Geometry check sheet. Reference: the model listing, model coordinates, mm. A direction names the side the tool comes from. Coordinates: 2 decimals unless noted, no trailing zeros. Order: outer loops, then holes, each group sorted by start corner. A loop starts at its lowest first (then second) coordinate and runs counter-clockwise, first axis right, second up. Notation, with made-up numbers: (59, 38) - (104, 38) arc R20 cw to (104, 55) - close; hole circle Ø6 at (-24, -33). An arc over 180 degrees is marked (long way). Use CSV: the item, a comma, the result in double quotes. Start each with the question number.
1) Sectioned sample at D-D, the plane y = -15. Record the cut outline in (x, z), and give its area (3 significant figures).
2) Sectioned sample at C-C, the plane y = -8. Record the cut outline in (x, z).
3) Sectioned sample at A-A, the plane y = 10. Record the cut outline in (x, z), and give its area (3 significant figures).
4) Tool access check on faces 5 (the cylindrical face through (24.305, -15.867, 11.014)), 6 (the flat face through (33, -10, 11)), 7 (the flat face through (0, -10, 11)). Record the directions out of +Z, -Z, +X, -X, +Y, -Y that give a thin tool (end or side, any length) a straight path to the whole face; none if there is none.
5) Depth check by flat-ended pin: P1, Ø6, axis at x = -10, z = 6, coming from the +Y side; P2, Ø1, axis at x = 35.5, z = 11.5, coming from the +Y side; P3, Ø5, axis at x = -10, z = 6, coming from the -Y side; P4, Ø3.5, axis at x = 25, y = 10, coming from the -Z side. Enter the tip coordinate at first touch or a pass-through.
6) Sectioned sample at B-B, the plane x = -10. Record the cut outline in (y, z), and give its area (3 significant figures).
7) Draft check along X on faces 1 (the flat face through (20, 0, 10)), 2 (the cylindrical face through (36.038, -13.004, 9.972)), 3 (the flat face through (0, 10, 5)), 4 (the flat face through (30, 10, 12)). Enter one of: released by +X, released by -X, zero draft, split by the parting line, or undercut.
8) Thickness scan on probe 1 along X at (y, z) = (10, 3.4); probe 2 along Y at (x, z) = (10, 1.45); probe 3 along X at (y, z) = (10, 7.6). Record the ranges inside material, lowest first. Write a range as [from, to].
from build123d import *

# Parameters (mm, degrees)
SKETCH_R                       = 2.25
PAD_DEPTH                      = 12
POCKET_DEPTH                   = 2
SKETCH002_R                    = 2.25
POCKET002_DEPTH                = 20.001
PART_MIRRORING_PLACEMENT_ANGLE = 180
SKETCH003_R                    = 3.75
POCKET003_DEPTH                = 5
SKETCH004_R                    = 3.75
POCKET004_DEPTH                = 10
SKETCH005_R                    = 3
POCKET005_DEPTH                = 8


with BuildPart() as pocket002:
    # Sketch → Pad (new body)
    with BuildSketch(Plane.XY):
        Polygon((0, -20), (40, -20), (40, 20), (-20, 20), (-20, 0), (0, 0), align=None)
        with Locations((15, 8)):
            Circle(SKETCH_R, mode=Mode.SUBTRACT)
        with Locations((10, -10)):
            Circle(SKETCH_R, mode=Mode.SUBTRACT)
        with Locations((35, 15)):
            Circle(SKETCH_R, mode=Mode.SUBTRACT)
        with Locations((25, -10)):
            Circle(SKETCH_R, mode=Mode.SUBTRACT)
    extrude(amount=PAD_DEPTH)

    # Sketch001 → Pocket (cut)
    with BuildSketch(Plane.XY.offset(12)):
        with BuildLine():
            Line((46, 10), (26, 10))
            ThreePointArc((26, 10), (22.778175, 17.778175), (15, 21))
            Line((15, 21), (0, 21))
            Line((0, 21), (0, -23))
            Line((0, -23), (46, -23))
            Line((46, -23), (46, -12))
            Line((25.382674, -13.981653), (46, -12))
            ThreePointArc((25.382674, -6.018347), (21, -10), (25.382674, -13.981653))
            Line((25.382674, -6.018347), (46, -8))
            Line((46, -8), (46, 10))
        make_face()
    extrude(amount=-POCKET_DEPTH, mode=Mode.SUBTRACT)

    # Sketch002 → Pocket002 (cut, through all)
    with BuildSketch(Plane.XZ):
        with Locations((-10, 6)):
            Circle(SKETCH002_R)
    extrude(amount=-POCKET002_DEPTH, mode=Mode.SUBTRACT)


with BuildPart() as pocket005:
    # Part__Mirroring: instance of Pocket002
    add(pocket002.part.mirror(Plane(origin=(0, 0, 0), x_dir=(0, 1, 0), z_dir=(0, 0, 1))))


with BuildPart() as pocket005_1:
    # Part__Mirroring placement: moved
    add(pocket005.part.rotate(Axis((0, 0, 0), (1, 0, 0)), PART_MIRRORING_PLACEMENT_ANGLE))

    # Sketch003 → Pocket003 (cut)
    with BuildSketch(Plane(origin=(0, 0, 0), x_dir=(1, 0, 0), z_dir=(0, 0, -1))):
        with Locations((10, -10)):
            Circle(SKETCH003_R)
        with Locations((25, -10)):
            Circle(SKETCH003_R)
    extrude(amount=-POCKET003_DEPTH, mode=Mode.SUBTRACT)

    # Sketch004 → Pocket004 (cut)
    with BuildSketch(Plane(origin=(0, -20, 0), x_dir=(-1, 0, 0), z_dir=(0, -1, 0))):
        with Locations((10, -6)):
            Circle(SKETCH004_R)
    extrude(amount=-POCKET004_DEPTH, mode=Mode.SUBTRACT)

    # Sketch005 → Pocket005 (cut)
    with BuildSketch(Plane(origin=(0, 0, 0), x_dir=(1, 0, 0), z_dir=(0, 0, -1))):
        with Locations((35, 15)):
            Circle(SKETCH005_R)
    extrude(amount=-POCKET005_DEPTH, mode=Mode.SUBTRACT)


solid = pocket005_1.part
Evaluation:
1,outline,"(-20, 0) - (32, 0) - (32, 8) - (32.75, 8) - (32.75, 12) - (24.8, 12) - (24.8, 10) - (0, 10) - (0, 12) - (-20, 12) - close; (37.25, 8) - (38, 8) - (38, 0) - (40, 0) - (40, 12) - (37.25, 12) - close; hole circle Ø7.5 at (-10, 6)"
1,area,"560 mm²"
2,outline,"(-20, 0) - (12.75, 0) - (12.75, 10) - (0, 10) - (0, 12) - (-20, 12) - close; (17.25, 0) - (40, 0) - (40, 10) - (17.25, 10) - close; hole circle Ø4.5 at (-10, 6)"
3,outline,"(0, 0) - (6.25, 0) - (6.25, 5) - (7.75, 5) - (7.75, 10) - (0, 10) - close; (12.25, 5) - (13.75, 5) - (13.75, 0) - (21.25, 0) - (21.25, 5) - (22.75, 5) - (22.75, 12) - (21, 12) - (21, 10) - (12.25, 10) - close; (27.25, 5) - (28.75, 5) - (28.75, 0) - (40, 0) - (40, 12) - (27.25, 12) - close"
3,area,"309 mm²"
4,face 5,"+Z"
4,face 6,"+Z, +X"
4,face 7,"+Z, +Y, -Y"
5,P1,"y = 0"
5,P2,"y = 13.06"
5,P3,"y = -10"
5,P4,"through"
6,outline,"(-20, 0) - (0, 0) - (0, 3.75) - (-10, 3.75) - (-10, 2.25) - (-20, 2.25) - close; (-20, 9.75) - (-10, 9.75) - (-10, 8.25) - (0, 8.25) - (0, 12) - (-20, 12) - close"
6,area,"120 mm²"
7,face 1,"undercut"
7,face 2,"undercut"
7,face 3,"released by -X"
7,face 4,"zero draft"
8,probe 1,"[0, 6.25], [13.75, 21.25], [28.75, 40]"
8,probe 2,"[-20, 6.25], [13.75, 20]"
8,probe 3,"[0, 7.75], [12.25, 22.75], [27.25, 40]"
